Design review of the part built by this model. Coordinates are the model's own, in mm. A direction names the side the tool comes from. Coordinates: 2 decimals unless noted, no trailing zeros. Loops run counter-clockwise (first coordinate to the right, second up) from the corner with the lowest first, then second, coordinate; pieces in that order, holes last. Notation, with made-up numbers: (-12, 54) - (44, 54) arc R7 cw to (44, 60) - close; hole circle Ø7 at (-18, 63). An arc over 180 degrees is marked (long way). Use one line per item in the form item = value. Start each with the question number.
(1) Tool access review of faces 1 (the face through (5, 11.402, 4)), 2 (the face through (5, -16, 0)): name each direction out of +Z, -Z, +X, -X, +Y, -Y from which nothing blocks a thin tool from reaching the whole face with its end or side.
(2) Add section B-B (x = 2.5). State the section outline as (y, z) points.
(3) For L1, parallel to Y at x = 6.75, z = 7.75; L2, parallel to Y at x = 7.5, z = 18; L3, parallel to Z at x = 5, y = 5.5, list the stretches that pass through material, from the lowest coordinate up.
(4) Add section D-D (y = -9). State the section outline as (x, z) points, plus the area to 3 significant figures.
(5) Clearance check with flat-ended pins moving along their axes: pin 1 Ø4 at (x, z) = (6.5, 20.5) entering from +Y; pin 2 Ø1 at (x, y) = (2, 7.5) entering from -Z. State where each tip first meets the part, or that it passes through.
(6) Add section A-A (z = 4). State the section outline as (x, y) points.
(7) Add section C-C (z = 14). State the section outline as (x, y) points.
(8) The part is to be moulded in two halves that separate along Y. For faces 3 (the face through (5, -11.402, 4)), 4 (the face through (10, -4, 20)), 5 (the face through (4.93, -10.009, 22.335)), say which applies: pulls with the +Y half, pulls with the -Y half, needs draft (parallel to the pull), parting line crosses it, or undercut.
```python
from build123d import *

# Parameters (mm, degrees)
PAD_DEPTH = 10


with BuildPart() as part:
    # Sketch → Pad (new body)
    with BuildSketch(Plane.YZ):
        with BuildLine():
            Line((11.40163, 0), (19.740902, 0))
            Line((19.740902, 0), (19.740902, 17.47224))
            Line((19.740902, 17.47224), (0, 27.335573))
            Line((0, 27.335573), (0, 20.068824))
            ThreePointArc((11.40163, 8.667194), (8.06217, 16.729364), (0, 20.068824))
            Line((11.40163, 0), (11.40163, 8.667194))
        make_face()
    pad = extrude(amount=PAD_DEPTH)

    # Mirrored: Pad across Sketch V_Axis
    add(pad.mirror(Plane(origin=(0, 0, 0), x_dir=(1, 0, 0), z_dir=(0, 1, 0))))


solid = part.part
```
Computed values:
q1.face_1 = -Z, +X, -X
q1.face_2 = -Z, +X, -X, +Y, -Y
q2.outline = (-19.74, 0) - (-11.4, 0) - (-11.4, 8.67) arc R11.4 cw to (11.4, 8.67) - (11.4, 0) - (19.74, 0) - (19.74, 17.47) - (0, 27.34) - (-19.74, 17.47) - close
q3.L1 = -19.74 to -11.4, 11.4 to 19.74
q3.L2 = -18.68 to -6.55, 6.55 to 18.68
q3.L3 = 18.65 to 24.59
q4.outline = (0, 15.67) - (10, 15.67) - (10, 22.84) - (0, 22.84) - close
q4.area = 71.7 mm^2
q5.pin_1 = 17.68
q5.pin_2 = 16.79
q6.outline = (0, -19.74) - (10, -19.74) - (10, -11.4) - (0, -11.4) - close; (0, 11.4) - (10, 11.4) - (10, 19.74) - (0, 19.74) - close
q7.outline = (0, -19.74) - (10, -19.74) - (10, -10.08) - (0, -10.08) - close; (0, 10.08) - (10, 10.08) - (10, 19.74) - (0, 19.74) - close
q8.face_3 = undercut
q8.face_4 = needs draft
q8.face_5 = pulls with the -Y half
